```python
from build123d import *

# Parameters (mm, degrees)
SKETCH_1_W          = 15
SKETCH_1_H          = 15
SKETCH_1_R          = 2.5
EXTRUDE_1_DEPTH     = 5
SKETCH_1_3_W        = 15
SKETCH_1_3_H        = 5
EXTRUDE_2_DEPTH     = 15
EXTRUDE_3_DEPTH     = 20
CUT_EXTRUDE_1_DEPTH = 20
SKETCH_3_W          = 10
SKETCH_3_H          = 10
CUT_EXTRUDE_2_DEPTH = 20
FILLET_1_R          = 10
SCALE_1_SCALE       = 0.2


with BuildPart() as part:
    # 草圖1 → 填料-伸長1 (new body)
    with BuildSketch(Plane(origin=(0, 0, 0), x_dir=(1, 0, 0), z_dir=(0, 1, 0))):
        with Locations((10, -2.5)):
            Rectangle(SKETCH_1_W, SKETCH_1_H)
        with Locations((10, -2.5)):
            Circle(SKETCH_1_R, mode=Mode.SUBTRACT)
    extrude(amount=EXTRUDE_1_DEPTH)

    # 草圖1<3> → 填料-伸長2 (add)
    with BuildSketch(Plane(origin=(0, 0, 0), x_dir=(1, 0, 0), z_dir=(0, 1, 0))):
        with Locations((10, 7.5)):
            Rectangle(SKETCH_1_3_W, SKETCH_1_3_H)
    extrude(amount=EXTRUDE_2_DEPTH)

    # 草圖1<4> → 填料-伸長3 (add)
    with BuildSketch(Plane(origin=(0, 0, 0), x_dir=(1, 0, 0), z_dir=(0, 1, 0))):
        Polygon((-17.5, 10), (-17.5, -10), (2.5, -10), (2.5, 5), (2.5, 10), align=None)
    extrude(amount=EXTRUDE_3_DEPTH)

    # 草圖2 → 除料-伸長1 (cut)
    with BuildSketch(Plane(origin=(2.5, 0, 0), x_dir=(0, 0, -1), z_dir=(1, 0, 0))):
        Polygon((-10, 5), (0, 20), (-10, 20), align=None)
    extrude(amount=-CUT_EXTRUDE_1_DEPTH, mode=Mode.SUBTRACT)

    # 草圖3 → 除料-伸長2 (cut)
    with BuildSketch(Plane(origin=(0, 0, -10), x_dir=(-1, 0, 0), z_dir=(0, 0, -1))):
        with Locations((7.5, 15)):
            Rectangle(SKETCH_3_W, SKETCH_3_H)
    extrude(amount=-CUT_EXTRUDE_2_DEPTH, mode=Mode.SUBTRACT)

    # 圓角1
    fillet_1_edges = [part.edges().sort_by_distance(p)[0] for p in [
        (17.5, 15, -7.5),
    ]]
    fillet(fillet_1_edges, radius=FILLET_1_R)


with BuildPart() as part_1:
    # 縮放比例1: scaled about (-2.616743612, 6.613370919, -1.498562555)
    add(part.part.scale(SCALE_1_SCALE).moved(Location((-2.09339489, 5.290696735, -1.198850044))))


solid = part_1.part
```
Here's how the part is built. I have some questions about the finished solid (model axes, mm). A direction names the side the tool comes from. Coordinates: 2 decimals unless noted, no trailing zeros. Order: outer loops, then holes, each group sorted by start corner. A loop starts at its lowest first (then second) coordinate and runs counter-clockwise, first axis right, second up. Notation, with made-up numbers: (31, -10) - (58, -10) arc R30 cw to (58, 27) - close; hole circle Ø6 at (-28, -5.5). An arc over 180 degrees is marked (long way). One line per question, with ' | ' between items. Start each with the question number.
1. Which directions (+Z, -Z, +X, -X, +Y, -Y) give clear straight access to the entire face, cutting with the end or side of a thin tool? Please do faces 4 (the flat face through (-2, 9.291, -2)), 5 (the flat face through (-1, 8.291, -3)), 6 (the flat face through (-2.593, 8, -2)), 7 (the flat face through (-2, 6, 0.801)), 8 (the flat face through (0, 7, -2.199)).
2. I'm going to push flat-ended pins straight in: pin 1 Ø2 at (x, y) = (-3.5, 8) entering from +Z; pin 2 Ø1 at (x, y) = (-0.5, 7) entering from +Z; pin 3 Ø1.1 at (x, z) = (-1, -2.5) entering from +Y. Where does each tip first touch, or does it pass through?
3. If we section it at B-B (y = 9.05): Write out the boundary of the cut face in (x, z).
4. Please list where these lines run through material, in increasing order: line 1 along X through (y, z) = (8.9, -2.1); line 2 along Y through (x, z) = (-3, -1.9); line 3 along X through (y, z) = (6.5, -1.55). Write a range as [from, to].
5. If we section it at C-C (z = -1.6): Write out the boundary of the cut face in (x, y).
6. If we mould it in two halves opening along Z, with no side actions, what happens to faces 1 (the cylindrical face through (-0.158, 5.784, -1.195)), 2 (the flat face through (-3.57, 7.1, 0.26)), 3 (the flat face through (-2, 5.291, -1))? For each: released by +Z, released by -Z, zero draft, split by the parting line, or undercut.
7. If we section it at D-D (x = -0.25): Write out the boundary of the cut face in (y, z).
8. If we section it at A-A (z = -0.35): Write out the boundary of the cut face in (x, y), and give its area (3 significant figures).
Model answer:
1) face 4: +Z, -Z, +X, -X, +Y | face 5: +Z, -Z, +X, +Y | face 6: +Z, -Z, +Y | face 7: +Z, +X, -X, +Y, -Y | face 8: +Z, +X, +Y
2) pin 1: stops at z = 0.33 | pin 2: stops at z = -2.2 | pin 3: stops at y = 8.29
3) outline: (-5.59, -3.2) - (-4.59, -3.2) - (-4.59, -1.04) - (-5.59, -1.04) - close; (-2.59, -3.2) - (-1.59, -3.2) - (-1.59, -1.04) - (-2.59, -1.04) - close
4) line 1: x = [-5.59, -4.59], [-2.59, -1.59] | line 2: y = [5.29, 7.29] | line 3: x = [-5.59, -1.59]
5) outline: (-5.59, 5.29) - (1.41, 5.29) - (1.41, 6.29) - (-1.59, 6.29) - (-1.59, 9.29) - (-2.59, 9.29) - (-2.59, 7.29) - (-4.59, 7.29) - (-4.59, 9.29) - (-5.59, 9.29) - close
6) face 1: undercut | face 2: released by +Z | face 3: zero draft
7) outline: (5.29, -3.2) - (8.26, -3.2) - (8.26, -2.2) - (6.29, -2.2) - (6.29, -1.17) - (5.29, -1.17) - close; (5.29, -0.22) - (6.29, -0.22) - (6.29, 0.8) - (5.29, 0.8) - close
8) outline: (-5.59, 5.29) - (-0.45, 5.29) - (-0.45, 6.29) - (-1.59, 6.29) - (-1.59, 8.02) - (-2.59, 8.02) - (-2.59, 7.29) - (-4.59, 7.29) - (-4.59, 8.02) - (-5.59, 8.02) - close; (0.26, 5.29) - (1.41, 5.29) - (1.41, 6.29) - (0.26, 6.29) - close | area: 11.7 mm²
